Answer from the drawing. Dimensions are ordinates in mm from the lowest x, y and z of the part. A direction names the side the tool comes from. Round coordinates to 2 decimals unless told otherwise and drop trailing zeros. Write each loop counter-clockwise with the first axis right and the second up, starting at its lowest first coordinate (ties: lowest second). Pieces come first, ordered by that corner, then holes. Notation, with made-up numbers: (-28.5, -1) - (8.5, -1) arc R25 cw to (8.5, 30) - close; hole circle Ø1 at (-31, -21.5). An arc over 180 degrees is marked (long way). Answer in a Markdown table with one row per item.
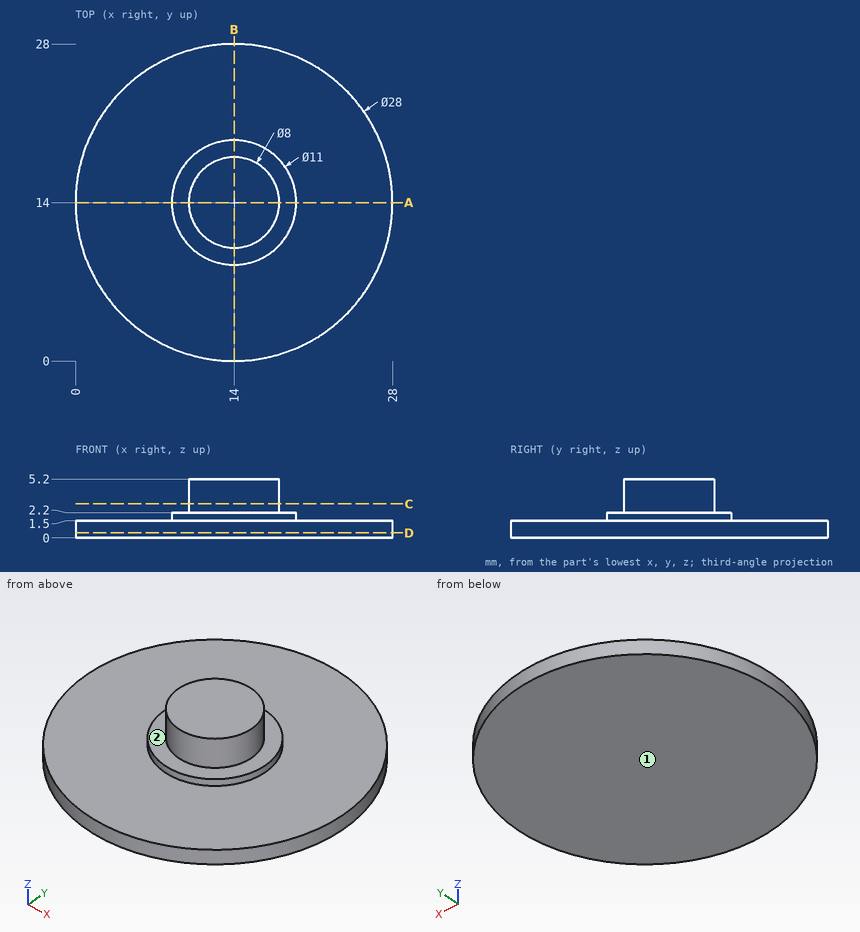
(1) Section D-D (z = 0.45) is taken. Give the vertices of the cut face in (x, y), and give its area (3 significant figures).
Checked values:
| item | result |
|---|---|
| outline | circle Ø28 at (14, 14) |
| area | 616 mm2 |
(2) Flat-ended cylindrical pins translate along their axes: pin 1 (1.5 mm diameter, centred on x = 20.5, z = 2, fed in from -Y); pin 2 (6 mm diameter, centred on x = 10, y = 9, fed in from -Z); pin 3 (3 mm diameter, centred on y = 4.5, z = 1.5, fed in from +X). Find the tip coordinate at first contact, or state that the pin passes through.
Checked values:
| item | result |
|---|---|
| pin 1 | stops at y = 1.32 |
| pin 2 | stops at z = 0 |
| pin 3 | stops at x = 25.49 |
(3) Find the intervals of material crossed by line 1 (Y direction, x = 14.25, z = 1.4); line 2 (Z direction, x = 18, y = 4.25); line 3 (X direction, y = 22.25, z = 1.25), in increasing order.
Checked values:
| item | result |
|---|---|
| line 1 | y = 0 to 28 |
| line 2 | z = 0 to 1.5 |
| line 3 | x = 2.69 to 25.31 |
(4) Section A-A (y = 14) is taken. Give the vertices of the cut face in (x, z), and give its area (3 significant figures).
Checked values:
| item | result |
|---|---|
| outline | (0, 0) - (28, 0) - (28, 1.5) - (19.5, 1.5) - (19.5, 2.2) - (18, 2.2) - (18, 5.2) - (10, 5.2) - (10, 2.2) - (8.5, 2.2) - (8.5, 1.5) - (0, 1.5) - close |
| area | 73.7 mm2 |
(5) Section C-C (z = 3) is taken. Give the vertices of the cut face in (x, y), and give its area (3 significant figures).
Checked values:
| item | result |
|---|---|
| outline | circle Ø8 at (14, 14) |
| area | 50.3 mm2 |
(6) For the marked faces 1 and 2, determine the directions among +Z, -Z, +X, -X, +Y, -Y from which every point of the face is accessible in a straight line to the end or side of a thin tool.
Checked values:
| item | result |
|---|---|
| face 1 | -Z, +X, -X, +Y, -Y |
| face 2 | +Z |
